The listing builds one solid part. Answer for the finished solid, in the listing's coordinates (mm). A direction names the side the tool comes from. Coordinates: 2 decimals unless noted, no trailing zeros. Order: outer loops, then holes, each group sorted by start corner. A loop starts at its lowest first (then second) coordinate and runs counter-clockwise, first axis right, second up. Notation, with made-up numbers: (37.5, -25) -> (55.5, -25) arc R17 ccw to (55.5, -18) -> close; hole circle Ø10 at (-30, 52). An arc over 180 degrees is marked (long way). Answer in a Markdown table with one row per item. Add a question column.
```python
from build123d import *

# Parameters (mm, degrees)
SKETCH_1_R      = 1.75
EXTRUDE_1_DEPTH = 5


with BuildPart() as part:
    # 草图1 → 凸台-拉伸1 (new body)
    with BuildSketch(Plane(origin=(0, 0, 0), x_dir=(1, 0, 0), z_dir=(0, 1, 0))):
        with BuildLine():
            Line((0, 5.5), (0, -5.5))
            ThreePointArc((0, -5.5), (0.585786438, -6.914213562), (2, -7.5))
            Line((2, -7.5), (43, -7.5))
            ThreePointArc((43, -7.5), (44.414213562, -6.914213562), (45, -5.5))
            Line((45, -5.5), (45, 5.5))
            ThreePointArc((45, 5.5), (44.414213562, 6.914213562), (43, 7.5))
            Line((43, 7.5), (2, 7.5))
            ThreePointArc((2, 7.5), (0.585786438, 6.914213562), (0, 5.5))
        make_face()
        with Locations((4, -2.5)):
            Circle(SKETCH_1_R, mode=Mode.SUBTRACT)
        with Locations((11, 2.5)):
            Circle(SKETCH_1_R, mode=Mode.SUBTRACT)
        with BuildLine():
            Line((30.028060952, -2), (40, -2))
            ThreePointArc((40, -2), (42, 3.9373e-05), (40, 2))
            Line((40, 2), (29.99998029, 1.999803136))
            ThreePointArc((29.99998029, 1.999803136), (28.000049288, -0.014237539), (30.028060952, -2))
        make_face(mode=Mode.SUBTRACT)
    extrude(amount=EXTRUDE_1_DEPTH)


solid = part.part
```
Q1. A cutting plane is placed at A-A (z = 2.5). Determine the outline of the cut face in (x, y).
Q2. Given pin 1 (4 mm diameter, centred on x = 11, z = -2.5, fed in from -Y), flat-ended and moving along its own axis, determine where the tip first touches the part or whether it passes through.
Q3. A cutting plane is placed at C-C (x = 11). Determine the outline of the cut face in (y, z), then the cut area to 3 significant figures.
Q4. For faces 1 (the face through (35, 2, 2)), 2 (the face through (0.57, 2.46, 6.9)), determine the directions among +Z, -Z, +X, -X, +Y, -Y from which every point of the face is accessible in a straight line to the end or side of a thin tool.
Q5. Straight lines are drawn through the part: line 1 (X direction, y = 3.1, z = -2.5); line 2 (Z direction, x = 11, y = 3.15); line 3 (Z direction, x = 4, y = 3.7). For each, find the intervals that lie inside material, in ascending order.
Q6. A cutting plane is placed at B-B (y = 3.4). Determine the outline of the cut face in (x, z).
Q7. Determine the mould class of faces 3 (the face through (23, 2, -7.5)), 4 (the face through (28, 2, 0)), 5 (the face through (22, 5, 0)), 6 (the face through (12.617, 2.465, -1.83)) for opening direction Z: +Z half, -Z half, draft (parallel to the pull), parting line (faces both ways), or undercut.
Returned:
| question | item | result |
|---|---|---|
| 1 | outline | (0, 0) -> (2.25, 0) -> (2.25, 5) -> (0, 5) -> close; (5.75, 0) -> (45, 0) -> (45, 5) -> (5.75, 5) -> close |
| 2 | pin 1 | stops at y = 0 |
| 3 | outline | (0, -7.5) -> (5, -7.5) -> (5, -4.25) -> (0, -4.25) -> close; (0, -0.75) -> (5, -0.75) -> (5, 7.5) -> (0, 7.5) -> close |
| 3 | area | 57.5 mm² |
| 4 | face 1 | +Y, -Y |
| 4 | face 2 | +Z, -X, +Y, -Y |
| 5 | line 1 | x = 0 to 9.25, 12.75 to 45 |
| 5 | line 2 | z = -7.5 to -4.25, -0.75 to 7.5 |
| 5 | line 3 | z = -7.5 to 0.75, 4.25 to 7.5 |
| 6 | outline | (0, -5.5) arc R2 ccw to (2, -7.5) -> (43, -7.5) arc R2 ccw to (45, -5.5) -> (45, 5.5) arc R2 ccw to (43, 7.5) -> (2, 7.5) arc R2 ccw to (0, 5.5) -> close; hole circle Ø3.5 at (4, 2.5); hole circle Ø3.5 at (11, -2.5); hole (30, -2) -> (40, -2) arc R2 ccw to (40, 2) -> (30.03, 2) arc R2 ccw (long way) to start |
| 7 | face 3 | -Z half |
| 7 | face 4 | undercut |
| 7 | face 5 | draft |
| 7 | face 6 | undercut |
